```python
from build123d import *

# Parameters (mm, degrees)
F1_DEPTH = 20
F2_T     = -2
F3_W     = 2
F3_H     = 1
F4_DEPTH = 26
F6_DEPTH = 30.001
F8_DEPTH = 2


# Not quite as in the source:
# - a shell that OpenCascade refuses in one call is made with other operations: the cavity is built on its own and cut out


with BuildPart() as f1:
    # F0 (on Right) → F1 (new body)
    with BuildSketch(Plane.YZ):
        Polygon((-13, -2), (-13, 0), (13, 0), (13, -2), (15, -2), (15, 20), (13, 20), (13, 22), (-13, 22), (-13, 20), (-15, 20), (-15, -2), align=None)
    extrude(amount=F1_DEPTH)

    # F2: a shell. OpenCascade refuses it in one call, so the cavity is built on its own and cut out:
    # the body offset inwards by the wall thickness, plus a prism from it out through each open face.
    f2_core = offset(f1.part, amount=F2_T, kind=Kind.INTERSECTION, mode=Mode.PRIVATE)
    f2_exits = [f2_core.faces().sort_by_distance(p)[0] for p in [
        (2, 0, 10.86087),
        (18, 0, 10.86087),
    ]]
    add(f2_core, mode=Mode.SUBTRACT)
    extrude(f2_exits, amount=-F2_T, mode=Mode.SUBTRACT)

    # F3 (on face) → F4 (join, through all)
    with BuildSketch(Plane.XZ.offset(-13)):
        with Locations((7, 2.5)):
            Rectangle(F3_W, F3_H)
        with Locations((13.2, 2.5)):
            Rectangle(F3_W, F3_H)
    extrude(amount=F4_DEPTH)

    # F5 (on face) → F6 (cut, through all)
    with BuildSketch(Plane.XZ.offset(15)):
        Polygon((16, 10), (10, 16), (4, 10), (10, 4), align=None)
    extrude(amount=-F6_DEPTH, mode=Mode.SUBTRACT)

    # F7 (on face) → F8 (cut, through all)
    with BuildSketch(Plane.XY.offset(22)):
        Polygon((17, 0), (10, 7), (3, 0), (10, -7), align=None)
    extrude(amount=-F8_DEPTH, mode=Mode.SUBTRACT)


solid = f1.part
```
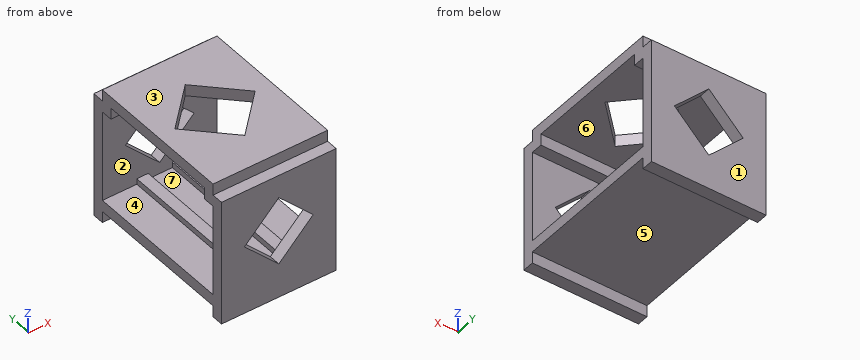
Verification items for the finished model (mm, model axes). Face numbers are marked on the shaded views. A direction names the side the tool comes from. Round coordinates to 2 decimals unless told otherwise and drop trailing zeros. Order: outer loops, then holes, each group sorted by start corner. A loop starts at its lowest first (then second) coordinate and runs counter-clockwise, first axis right, second up. Notation, with made-up numbers: (15.5, 54.5) -> (57.5, 54.5) arc R29 cw to (57.5, 75.5) -> close; hole circle Ø7 at (-30, -16.5). An arc over 180 degrees is marked (long way). Put each result on its own line as item: value. Start each with the question number.
(1) Section check C-C (y = -12). Enter the section's corners in (x, z), then the cut area to 3 significant figures.
(2) Draft check along Y on the marked faces 1, 2 and 3. Enter one of: +Y half, -Y half, draft (parallel to the pull), parting line (faces both ways), or undercut.
(3) Material ranges on line 1 along Y through (x, z) = (16, 7.5); line 2 along Y through (x, z) = (14.5, 19.5); line 3 along Z through (x, y) = (3.25, 8), recorded low to high.
(4) Tool access check on the marked faces 4, 5, 6 and 7. Record the directions out of +Z, -Z, +X, -X, +Y, -Y that give a thin tool (end or side, any length) a straight path to the whole face; none if there is none.
(5) Section check B-B (z = 8.5). Enter the section's corners in (x, y), then the cut area to 3 significant figures.
(6) Section check A-A (x = 5.5). State how many separate pieces and enclosed holes the cut face has, then the cut area to 3 significant figures.
(7) Depth check by flat-ended pin: pin 1 Ø1.6 at (x, y) = (9.5, -12) entering from -Z; pin 2 Ø0.8 at (y, z) = (-3, 2.5) entering from -X; pin 3 Ø2 at (x, y) = (7, -1.5) entering from +Z. Enter the tip coordinate at first touch or a pass-through.
(8) Section check D-D (y = -1). Enter the section's corners in (x, z).
Completed:
1. outline: (0, 0) -> (20, 0) -> (20, 2) -> (14.2, 2) -> (14.2, 3) -> (12.2, 3) -> (12.2, 2) -> (8, 2) -> (8, 3) -> (6, 3) -> (6, 2) -> (0, 2) -> close; (0, 18) -> (20, 18) -> (20, 22) -> (0, 22) -> close
1. area: 124 mm2
2. face 1: +Y half
2. face 2: undercut
2. face 3: draft
3. line 1: y = -15 to -13, 13 to 15
3. line 2: y = -15 to -11, 11 to 15
3. line 3: z = 0 to 2, 20 to 22
4. face 4: -X
4. face 5: -Z, +X, -X
4. face 6: +X, -X
4. face 7: none
5. outline: (0, -15) -> (5.5, -15) -> (5.5, -13) -> (0, -13) -> close; (0, 13) -> (5.5, 13) -> (5.5, 15) -> (0, 15) -> close; (14.5, -15) -> (20, -15) -> (20, -13) -> (14.5, -13) -> close; (14.5, 13) -> (20, 13) -> (20, 15) -> (14.5, 15) -> close
5. area: 44.0 mm2
6. separate pieces: 3
6. enclosed holes: 0
6. area: 178 mm2
7. pin 1: stops at z = 0
7. pin 2: stops at x = 6
7. pin 3: stops at z = 3
8. outline: (0, 0) -> (20, 0) -> (20, 2) -> (14.2, 2) -> (14.2, 3) -> (12.2, 3) -> (12.2, 2) -> (8, 2) -> (8, 3) -> (6, 3) -> (6, 2) -> (0, 2) -> close; (0, 20) -> (4, 20) -> (4, 22) -> (0, 22) -> close; (16, 20) -> (20, 20) -> (20, 22) -> (16, 22) -> close
